```python
from build123d import *

# Parameters (mm, degrees)
PAD008_DEPTH    = 9.7
POCKET002_DEPTH = 3.9
PAD009_DEPTH    = 7
SKETCH048_R     = 1.6
SKETCH048_R_2   = 1.3
POCKET030_DEPTH = 15.001
FILLET006_R     = 5
FILLET007_R     = 2
FILLET008_R     = 1


with BuildPart() as part:
    # Sketch045 → Pad008 (new body)
    with BuildSketch(Plane.XY):
        with BuildLine():
            Line((-7, 19), (0, 19))
            Line((0, 19), (0, 6.2))
            ThreePointArc((0, 6.2), (-6.2, 0), (0, -6.2))
            Line((0, -6.2), (0, -19))
            Line((0, -19), (-7, -19))
            Line((-7, -19), (-7, -9.1241437954))
            ThreePointArc((-7, 9.1241437954), (-11.5, 0), (-7, -9.1241437954))
            Line((-7, 9.1241437954), (-7, 19))
        make_face()
    extrude(amount=-PAD008_DEPTH)

    # Sketch046 → Pocket002 (cut)
    with BuildSketch(Plane.XY):
        with BuildLine():
            Line((0, 11.5), (0, 6.2))
            ThreePointArc((0, 6.2), (-6.2, 0), (0, -6.2))
            Line((0, -6.2), (0, -11.5))
            ThreePointArc((0, 11.5), (-11.5, 0), (0, -11.5))
        make_face()
    extrude(amount=-POCKET002_DEPTH, mode=Mode.SUBTRACT)

    # Sketch047 → Pad009 (join)
    with BuildSketch(Plane.YZ.offset(-15)):
        with BuildLine():
            ThreePointArc((13.2003787824, -21.6), (0, -13.1), (-13.2003787824, -21.6))
            Line((-16.5, -21.6), (-13.2003787824, -21.6))
            Line((-16.5, -13.5843597113), (-16.5, -21.6))
            ThreePointArc((-12.75, -9.5921798557), (-15.4154759474, -10.8457469238), (-16.5, -13.5843597113))
            ThreePointArc((-12.75, -9.5921798557), (-10.0845240526, -8.3386127875), (-9, -5.6))
            Line((-9, -5.6), (-9, -3.6))
            Line((-9, -3.6), (9, -3.6))
            Line((9, -3.6), (9, -5.6))
            ThreePointArc((9, -5.6), (10.0845240526, -8.3386127875), (12.75, -9.5921798557))
            ThreePointArc((16.5, -13.5843597113), (15.4154759474, -10.8457469238), (12.75, -9.5921798557))
            Line((16.5, -13.5843597113), (16.5, -21.6))
            Line((16.5, -21.6), (13.2003787824, -21.6))
        make_face()
    extrude(amount=PAD009_DEPTH)

    # Sketch048 → Pocket030 (cut, through all)
    with BuildSketch(Plane.YZ):
        with Locations((-14.75, -4.8)):
            Circle(SKETCH048_R)
        with Locations((14.75, -4.8)):
            Circle(SKETCH048_R)
        with Locations((-12, -15.3)):
            Circle(SKETCH048_R_2)
        with Locations((12, -15.3)):
            Circle(SKETCH048_R_2)
    extrude(amount=-POCKET030_DEPTH, mode=Mode.SUBTRACT)

    # Fillet006
    fillet006_edges = [part.edges().sort_by_distance(p)[0] for p in [
        (-3.5, 19, -9.7),
        (-3.5, -19, -9.7),
    ]]
    fillet(fillet006_edges, radius=FILLET006_R)

    # Fillet007
    fillet007_edges = [part.edges().sort_by_distance(p)[0] for p in [
        (-11.5, -13.200379, -21.6),
        (-11.5, -16.5, -21.6),
        (-11.5, 13.200379, -21.6),
        (-11.5, 16.5, -21.6),
    ]]
    fillet(fillet007_edges, radius=FILLET007_R)

    # Fillet008
    fillet008_edges = [part.edges().sort_by_distance(p)[0] for p in [
        (-6.2, 0, -3.9),
        (-6.2, 0, -9.7),
        (0, -8.85, -3.9),
        (0, -10.1, -9.7),
        (0, 8.85, -3.9),
        (0, 10.1, -9.7),
    ]]
    fillet(fillet008_edges, radius=FILLET008_R)


solid = part.part
```
The model under review builds one solid part; all positions refer to its coordinate system, in mm. A direction names the side the tool comes from. Round coordinates to 2 decimals unless told otherwise and drop trailing zeros. Order: outer loops, then holes, each group sorted by start corner. A loop starts at its lowest first (then second) coordinate and runs counter-clockwise, first axis right, second up. Notation, with made-up numbers: M -8,7.25 L 49,7.25 A25 cw 49,42.25 Z; hole C 84.25,74 d5. An arc over 180 degrees is marked long. Use a Markdown table: item, result.
1) Consider section A-A (y = 0). Write out the cut boundary in (x, z).
Report:
| item | result |
|---|---|
| outline | M -15,-13.1 L -8,-13.1 L -8,-9.7 L -7.2,-9.7 A1 ccw -6.2,-8.7 L -6.2,-4.9 A1 ccw -7.2,-3.9 L -8,-3.9 L -8,-3.6 L -15,-3.6 Z |
2) Tool access review of faces 1 (the face through (-12, 9, -5)), 2 (the face through (-3.646, 10.907, -1.871)), 3 (the face through (-6.2, 0.1, -6.8)), 4 (the face through (-11, 13, -21)): name each direction out of +Z, -Z, +X, -X, +Y, -Y from which nothing blocks a thin tool from reaching the whole face with its end or side.
Report:
| item | result |
|---|---|
| face 1 | +Z, -X, +Y |
| face 2 | +Z, +X |
| face 3 | +Z, -Z, +X |
| face 4 | -Z, +X, -X |
3) Consider section C-C (z = -15.3). Write out the cut boundary in (x, y).
Report:
| item | result |
|---|---|
| outline | M -15,-16.5 L -8,-16.5 L -8,-13.3 L -15,-13.3 Z; M -15,-10.7 L -8,-10.7 L -8,-7.68 L -15,-7.68 Z; M -15,7.68 L -8,7.68 L -8,10.7 L -15,10.7 Z; M -15,13.3 L -8,13.3 L -8,16.5 L -15,16.5 Z |
4) Consider section B-B (x = -10.5). Write out the cut boundary in (y, z).
Report:
| item | result |
|---|---|
| outline | M -16.5,-19.6 A2 ccw -14.5,-21.6 L -14.43,-21.6 A2 ccw -12.68,-20.57 A14.5 cw 12.68,-20.57 A2 ccw 14.43,-21.6 L 14.5,-21.6 A2 ccw 16.5,-19.6 L 16.5,-13.58 A4 ccw 12.75,-9.59 A4 cw 9,-5.6 L 9,-3.6 L -9,-3.6 L -9,-5.6 A4 cw -12.75,-9.59 A4 ccw -16.5,-13.58 Z; hole C -12,-15.3 d2.6; hole C 12,-15.3 d2.6 |
5) Draft analysis for pull direction Z (two halves, no side actions). For faces 5 (the face through (-4.04, -17.5, -8.27)), 6 (the face through (-12, -9, -5)), 7 (the face through (-11.5, -10.8, -15.8)), state which applies: released by +Z, released by -Z, zero draft, split by the parting line, or undercut.
Report:
| item | result |
|---|---|
| face 5 | released by -Z |
| face 6 | zero draft |
| face 7 | undercut |
6) Insertion check: pin 1 (8 mm diameter, centred on y = 16, z = -6.5, fed in from -X); pin 2 (3 mm diameter, centred on y = 12, z = -3, fed in from -X); pin 3 (5.5 mm diameter, centred on x = -3, y = 2, fed in from -Z); pin 4 (6.5 mm diameter, centred on x = -10.5, z = -16, fed in from -Y). Each pin has a flat end and moves straight along its axis. Give the tip position at first contact, or say it passes through.
Report:
| item | result |
|---|---|
| pin 1 | x = -15 |
| pin 2 | x = -7 |
| pin 3 | z = -9.24 |
| pin 4 | y = -16.5 |
7) Consider section D-D (z = -20). Write out the cut boundary in (x, y).
Report:
| item | result |
|---|---|
| outline | M -15,-16.46 L -8,-16.46 L -8,-12.35 L -15,-12.35 Z; M -15,12.35 L -8,12.35 L -8,16.46 L -15,16.46 Z |
8) Wall thickness on line 1 along Z through (x, y) = (-11.25, 12); line 2 along Y through (x, z) = (-1.5, -2); line 3 along Z through (x, y) = (-3.25, -16): over which ranges is each line inside the solid? List them lowest first. Write a range as [from, to].
Report:
| item | result |
|---|---|
| line 1 | [-19.46, -16.6], [-14, -9.47] |
| line 2 | [-19, -11.4], [11.4, 19] |
| line 3 | [-9.28, -5.8], [-3.8, 0] |
